from build123d import *

# Parameters (mm, degrees)
SKETCH_9688_R   = 1.55
SKETCH_9688_R_2 = 1.075
SKETCH_9688_W   = 13.4
SKETCH_9688_H   = 18.1
SKETCH_9688_R_3 = 1.3
SKETCH_9688_W_2 = 15.95
SKETCH_9688_H_2 = 15.5
PCB_DEPTH       = 1.6


with BuildPart() as part:
    # Sketch 9688 → 主结构-PCB最大范围-实际可以比这个小 (new body)
    with BuildSketch(Plane(origin=(0, 0, 0), x_dir=(1, 0, 0), z_dir=(0, 1, 0))):
        Polygon((3.75, 45), (6.5, 42.25), (6.5, 29.683072379), (6, 29.183072379), (-8.425, 29.183072379), (-10.425, 27.183072379), (-10.425, 11.824221247), (-22, 5.141391882), (-22, -23.812684418), (-9.65, -30.942960242), (-9.15, -31.231635377), (-9.15, -34.122764912), (-9.15, -60.451116293), (-12.65, -63.951116293), (-12.65, -69.046082783), (-9.15, -72.546082783), (-9.15, -75.200927376), (-4.100927376, -80.25), (4.100927376, -80.25), (9.65, -74.700927376), (9.65, -56.5), (8.4, -55.25), (8.4, -33.506128091), (11.45, -30.456128091), (11.45, 5.014466094), (8.2, 8.264466094), (8.2, 13.127500889), (18.25, 23.177500889), (18.25, 30.170693918), (18.25, 42.25), (21, 45), (21.35, 45), (24.85, 48.5), (24.85, 68.199999999), (22.1, 70.949999999), (-8.75, 70.949999999), (-11.5, 68.199999999), (-11.5, 49.5), (-7, 45), align=None)
        with Locations(Location((0, -76.75, 0), (0, 0, 270))):
            Circle(SKETCH_9688_R, mode=Mode.SUBTRACT)
        with BuildLine():
            Line((-4.100927376, -61.951116293), (-4.100927376, -58.5))
            Line((-4.100927376, -58.5), (-0.000927376, -58.5))
            Line((-0.000927376, -58.5), (0.000927376, -58.5))
            Line((0.000927376, -58.5), (4.100927376, -58.5))
            Line((4.100927376, -58.5), (4.100927376, -61.951116293))
            ThreePointArc((4.100927376, -61.951116293), (4.203440002, -62.198603667), (4.450927376, -62.301116293))
            Line((4.450927376, -62.301116293), (4.54842161, -62.301116293))
            ThreePointArc((4.54842161, -62.301116293), (7.376848734, -63.472689168), (8.54842161, -66.301116291))
            Line((8.54842161, -66.301116291), (8.54842161, -66.696082786))
            ThreePointArc((8.54842161, -66.696082786), (7.376848734, -69.524509909), (4.54842161, -70.696082783))
            Line((4.54842161, -70.696082783), (4.450927376, -70.696082783))
            ThreePointArc((4.450927376, -70.696082783), (4.203440002, -70.79859541), (4.100927376, -71.046082783))
            Line((4.100927376, -71.046082783), (4.100927376, -74.497199077))
            Line((4.100927376, -74.497199077), (0.000927376, -74.497199077))
            Line((0.000927376, -74.497199077), (-0.000927376, -74.497199077))
            Line((-0.000927376, -74.497199077), (-4.100927376, -74.497199077))
            Line((-4.100927376, -74.497199077), (-4.100927376, -71.046082783))
            ThreePointArc((-4.100927376, -71.046082783), (-4.203440002, -70.79859541), (-4.450927376, -70.696082783))
            Line((-4.450927376, -70.696082783), (-4.54842161, -70.696082783))
            ThreePointArc((-4.54842161, -70.696082783), (-7.376848734, -69.524509909), (-8.54842161, -66.696082786))
            Line((-8.54842161, -66.696082786), (-8.54842161, -66.301116291))
            ThreePointArc((-8.54842161, -66.301116291), (-7.376848734, -63.472689168), (-4.54842161, -62.301116293))
            Line((-4.54842161, -62.301116293), (-4.450927376, -62.301116293))
            ThreePointArc((-4.450927376, -62.301116293), (-4.203440002, -62.198603667), (-4.100927376, -61.951116293))
        make_face(mode=Mode.SUBTRACT)
        with Locations(Location((0, -56.25, 0), (0, 0, 270))):
            Circle(SKETCH_9688_R, mode=Mode.SUBTRACT)
        with Locations(Location((-15.25, -15.25, 0), (0, 0, 270))):
            Circle(SKETCH_9688_R, mode=Mode.SUBTRACT)
        with Locations(Location((-12.75, -12.75, 0), (0, 0, 270))):
            Circle(SKETCH_9688_R_2, mode=Mode.SUBTRACT)
        with Locations(Location((-10, -10, 0), (0, 0, 270))):
            Circle(SKETCH_9688_R_2, mode=Mode.SUBTRACT)
        with BuildLine():
            Line((-8.95, -8.239318314), (-8.95, 3.966927621))
            Line((-8.95, 3.966927621), (8.95, 3.966927621))
            Line((8.95, 3.966927621), (8.95, -8.239318314))
            ThreePointArc((8.95, -8.239318314), (7.95, -10), (8.95, -11.760681686))
            Line((8.95, -11.760681686), (8.95, -27.933072379))
            Line((8.95, -27.933072379), (-8.95, -27.933072379))
            Line((-8.95, -27.933072379), (-8.95, -11.760681686))
            ThreePointArc((-8.95, -11.760681686), (-7.95, -10), (-8.95, -8.239318314))
        make_face(mode=Mode.SUBTRACT)
        with Locations(Location((10, -10, 0), (0, 0, 270))):
            Circle(SKETCH_9688_R_2, mode=Mode.SUBTRACT)
        with Locations((0, 18.383072379)):
            Rectangle(SKETCH_9688_W, SKETCH_9688_H, mode=Mode.SUBTRACT)
        with Locations(Location((3.8, 62.12002051, 0), (0, 0, 270))):
            Circle(SKETCH_9688_R_3, mode=Mode.SUBTRACT)
        with Locations(Location((19.5, 47.800000001, 0), (0, 0, 270))):
            Circle(SKETCH_9688_R_3, mode=Mode.SUBTRACT)
        with Locations((15.625, 58)):
            Rectangle(SKETCH_9688_W_2, SKETCH_9688_H_2, mode=Mode.SUBTRACT)
        with Locations(Location((19.5, 68.199999999, 0), (0, 0, 270))):
            Circle(SKETCH_9688_R_3, mode=Mode.SUBTRACT)
    extrude(amount=PCB_DEPTH)


solid = part.part
Here's how the part is built. I have some questions about the finished solid (model axes, mm). A direction names the side the tool comes from. Give positions to 0.01 mm unless a question says otherwise; leave off trailing zeros. Order: outer loops, then holes, each group sorted by start corner. A loop starts at its lowest first (then second) coordinate and runs counter-clockwise, first axis right, second up. Notation, with made-up numbers: (80.25, 40.25) -> (134.25, 40.25) arc R23 cw to (134.25, 48.25) -> close; hole circle Ø4 at (56.25, 83.5). An arc over 180 degrees is marked (long way). Use a Markdown table: item, result. Add a question column.
Item 1: If we mould it in two halves opening along X, with no side actions, what happens to faces 1 (the face through (0.466, 0.789, 57.728)), 2 (the face through (9.848, 0.789, -6.617)), 3 (the face through (-10.1, 0.8, -69.6))? For each: pulls with the +X half, pulls with the -X half, needs draft (parallel to the pull), parting line crosses it, or undercut.
Item 2: Will these pins go through, and if not, where does the flat tip stop? pin 1 (12 mm diameter, centred on x = 17, z = 63, fed in from -Y); pin 2 (0.8 mm diameter, centred on y = 0.5, z = -61, fed in from -X); pin 3 (0.5 mm diameter, centred on y = 1, z = 50, fed in from -X).
Item 3: I need wall thicknesses on line 1 (X direction, y = 1.2, z = 10) (3 decimals); line 2 (X direction, y = 0.9, z = 12.5); line 3 (X direction, y = 1.2, z = 66). Which ranges of each line are inside material? Lowest first, please.
Item 4: Imagine slicing it at D-D on z = 41. Please give me the cut outline in (x, y), plus the area to 3 significant figures.
Item 5: For faces 4 (the face through (-9, 1, -47)), 5 (the face through (9.904, 0.789, 32.002)), 6 (the face through (7.4, 0.8, 69.5)), which set-ups out of +Z, -Z, +X, -X, +Y, -Y let a thin tool reach every point of the face, with its end or its side?
Item 6: Imagine slicing it at B-B on z = 76.75. Please give me the cut outline in (x, y), plus the area to 3 significant figures.
Item 7: Imagine slicing it at A-A on x = 14.5. Please give me the cut outline in (y, z).
Item 8: Imagine slicing it at C-C on y = 0.3. Give the number of separate pieces and of enclosed holes in the cut face, plus the area to 3 significant figures.
Data:
| question | item | result |
|---|---|---|
| 1 | face 1 | undercut |
| 1 | face 2 | pulls with the +X half |
| 1 | face 3 | pulls with the -X half |
| 2 | pin 1 | passes through |
| 2 | pin 2 | stops at x = -11.5 |
| 2 | pin 3 | stops at x = -9.15 |
| 3 | line 1 | x = -22 to -11.075, -8.925 to -7.95, 7.95 to 8.925, 11.075 to 11.45 |
| 3 | line 2 | x = -22 to -13.8, -11.7 to -8.95, 8.95 to 11.45 |
| 3 | line 3 | x = -12.65 to -8.54, 8.54 to 9.65 |
| 4 | outline | (-9.15, 0) -> (8.4, 0) -> (8.4, 1.6) -> (-9.15, 1.6) -> close |
| 4 | area | 28.1 mm² |
| 5 | face 4 | -X, +Y, -Y |
| 5 | face 5 | +X, +Y, -Y |
| 5 | face 6 | +Y, -Y |
| 6 | outline | (-7.6, 0) -> (-1.55, 0) -> (-1.55, 1.6) -> (-7.6, 1.6) -> close; (1.55, 0) -> (7.6, 0) -> (7.6, 1.6) -> (1.55, 1.6) -> close |
| 6 | area | 19.4 mm² |
| 7 | outline | (0, -70.95) -> (1.6, -70.95) -> (1.6, -65.75) -> (0, -65.75) -> close; (0, -50.25) -> (1.6, -50.25) -> (1.6, -19.43) -> (0, -19.43) -> close |
| 8 | separate pieces | 1 |
| 8 | enclosed holes | 13 |
| 8 | area | 2,480 mm² |
